Autodesk Inventor part; units mm, degrees
ref_plane "YZ Plane" through (0, 0, 0) normal (1, 0, 0) x (0, 1, 0)
ref_plane "XZ Plane" through (0, 0, 0) normal (0, 1, 0) x (-1, 0, 0)
ref_plane "XY Plane" through (0, 0, 0) normal (0, 0, 1) x (1, 0, 0)
sketch "Sketch1" plane through (0, 0, 0) normal (0, 1, 0) x (-1, 0, 0)
  line L0 (6.3636, -25.4) -> (6.3636, 25.4)
  line L1 (-6.3364, 25.2915) -> (-6.3364, -25.2915)
  line L2 (-6.3364, -25.2915) -> (6.3636, 25.4) construction
  line L3 (6.3636, -25.4) -> (-6.3364, 25.2915) construction
  arc A0 (6.3636, 25.4) -> (-6.3364, 25.2915) centre (0.0131, 25.4) ccw
  arc A1 (-6.3364, -25.2915) -> (6.3636, -25.4) centre (0.0131, -25.4) ccw
  circle A2 centre (0.0131, 25.4) radius 1.5434
  point P0 (0, 0)
  dimension "d0" = 50.8
  dimension "d1" = 12.7
extrude "Extrusion1" add sketch "Sketch1" along normal blind 6.35
properties part number "Fixture_Lever"
Source: CAD feature listing. Evaluate the final solid. Frame: model axes, mm. Give positions to 0.01 mm unless a question says otherwise; leave off trailing zeros. Order: outer loops, then holes, each group sorted by start corner. A loop starts at its lowest first (then second) coordinate and runs counter-clockwise, first axis right, second up. Notation, with made-up numbers: (27, -21.5) -> (58, -21.5) arc R19 cw to (58, -5.5) -> close; hole circle Ø1 at (36.5, 71.25). An arc over 180 degrees is marked (long way). Use a Markdown table: item, result.
Q1. Pull-direction query (Z, two-part tool) for faces 1 (the face through (-0.725, 3.131, 26.769)), 2 (the face through (0, 0, 0)); classes: +Z half, -Z half, draft (parallel to the pull), parting line (faces both ways), or undercut.
A:
| item | result |
|---|---|
| face 1 | undercut |
| face 2 | draft |
Q2. Section B-B (x = -0.75). Return the cut outline in (y, z).
A:
| item | result |
|---|---|
| outline | (0, -31.71) -> (6.35, -31.71) -> (6.35, 24.04) -> (0, 24.04) -> close; (0, 26.76) -> (6.35, 26.76) -> (6.35, 31.71) -> (0, 31.71) -> close |
Q3. Section D-D (x = 4.5). Return the cut outline in (y, z), and give its area (3 significant figures).
A:
| item | result |
|---|---|
| outline | (0, -29.87) -> (6.35, -29.87) -> (6.35, 29.87) -> (0, 29.87) -> close |
| area | 379 mm^2 |
Q4. Material intervals for line 1 (Z direction, x = 0, y = 3.25); line 2 (Z direction, x = 1, y = 5.25); line 3 (Z direction, x = -4.5, y = 2.75), sorted ascending. Write a range as [from, to].
A:
| item | result |
|---|---|
| line 1 | [-31.75, 23.86], [26.94, 31.75] |
| line 2 | [-31.67, 24.24], [26.56, 31.67] |
| line 3 | [-29.89, 29.89] |
Q5. First-contact query: P1, Ø1, axis at x = -2, y = 3.5, coming from the -Z side. Flat tip, straight axial feed; report the tip coordinate or a pass-through.
A:
| item | result |
|---|---|
| P1 | z = -31.57 |
Q6. Section A-A (y = 1.5). Return the cut outline in (x, z), and give its area (3 significant figures).
A:
| item | result |
|---|---|
| outline | (-6.36, -25.4) arc R6.35 ccw (long way) to (6.34, -25.29) -> (6.34, 25.29) arc R6.35 ccw (long way) to (-6.36, 25.4) -> close; hole circle Ø3.09 at (-0.01, 25.4) |
| area | 764 mm^2 |
Q7. Section C-C (x = -3.75). Return the cut outline in (y, z), and give its area (3 significant figures).
A:
| item | result |
|---|---|
| outline | (0, -30.53) -> (6.35, -30.53) -> (6.35, 30.53) -> (0, 30.53) -> close |
| area | 388 mm^2 |
